Source: CAD feature listing. Evaluate the final solid. Frame: model axes, mm. A direction names the side the tool comes from. Give positions to 0.01 mm unless a question says otherwise; leave off trailing zeros. Order: outer loops, then holes, each group sorted by start corner. A loop starts at its lowest first (then second) coordinate and runs counter-clockwise, first axis right, second up. Notation, with made-up numbers: (43.5, 82) -> (78.5, 82) arc R18 ccw to (78.5, 100) -> close; hole circle Ø4 at (-27, 79.25). An arc over 180 degrees is marked (long way). Answer in a Markdown table with one row per item.
```python
from build123d import *

# Parameters (mm, degrees)
F0_R     = 38.1
F1_DEPTH = 25.4


with BuildPart() as f1:
    # F0 (on Front) → F1 (new body)
    with BuildSketch(Plane.XZ):
        with BuildLine():
            ThreePointArc((49.1988245643, 12.6536817364), (50.3981164721, 6.3772922205), (50.8, 0))
            ThreePointArc((50.8, 0), (50.3981164721, -6.3772922205), (49.1988245643, -12.6536817364))
            Line((49.1988245643, -12.6536817364), (49.5602090261, -13.2796179853))
            Line((49.5602090261, -13.2796179853), (72.5611820817, 0))
            Line((72.5611820817, 0), (49.5602090261, 13.2796179853))
            Line((49.5602090261, 13.2796179853), (49.1988245643, 12.6536817364))
        make_face()
        with BuildLine():
            ThreePointArc((48.9342727773, 13.641002447), (49.0690319755, 13.1480074912), (49.1988245643, 12.6536817364))
            Line((49.1988245643, 12.6536817364), (49.5602090261, 13.2796179853))
            Line((49.5602090261, 13.2796179853), (48.9342727773, 13.641002447))
        make_face()
        with BuildLine():
            Line((49.5602090261, -13.2796179853), (49.1988245643, -12.6536817364))
            ThreePointArc((49.1988245643, -12.6536817364), (49.0690319755, -13.1480074912), (48.9342727773, -13.641002447))
            Line((48.9342727773, -13.641002447), (49.5602090261, -13.2796179853))
        make_face()
        with BuildLine():
            ThreePointArc((36.2805910408, 35.5578221173), (43.9940905122, 25.4), (48.9342727773, 13.641002447))
            Line((48.9342727773, 13.641002447), (49.5602090261, 13.2796179853))
            Line((49.5602090261, 13.2796179853), (62.8398270114, 36.2805910408))
            Line((62.8398270114, 36.2805910408), (36.2805910408, 36.2805910408))
            Line((36.2805910408, 36.2805910408), (36.2805910408, 35.5578221173))
        make_face()
        with BuildLine():
            Line((49.5602090261, -13.2796179853), (48.9342727773, -13.641002447))
            ThreePointArc((48.9342727773, -13.641002447), (43.9940905122, -25.4), (36.2805910408, -35.5578221173))
            Line((36.2805910408, -35.5578221173), (36.2805910408, -36.2805910408))
            Line((36.2805910408, -36.2805910408), (62.8398270114, -36.2805910408))
            Line((62.8398270114, -36.2805910408), (49.5602090261, -13.2796179853))
        make_face()
        with BuildLine():
            ThreePointArc((35.5578221173, 36.2805910408), (35.9210244843, 35.9210244843), (36.2805910408, 35.5578221173))
            Line((36.2805910408, 35.5578221173), (36.2805910408, 36.2805910408))
            Line((36.2805910408, 36.2805910408), (35.5578221173, 36.2805910408))
        make_face()
        with BuildLine():
            Line((36.2805910408, -36.2805910408), (36.2805910408, -35.5578221173))
            ThreePointArc((36.2805910408, -35.5578221173), (35.9210244843, -35.9210244843), (35.5578221173, -36.2805910408))
            Line((35.5578221173, -36.2805910408), (36.2805910408, -36.2805910408))
        make_face()
        with BuildLine():
            ThreePointArc((13.641002447, 48.9342727773), (25.4, 43.9940905122), (35.5578221173, 36.2805910408))
            Line((35.5578221173, 36.2805910408), (36.2805910408, 36.2805910408))
            Line((36.2805910408, 36.2805910408), (36.2805910408, 62.8398270114))
            Line((36.2805910408, 62.8398270114), (13.2796179853, 49.5602090261))
            Line((13.2796179853, 49.5602090261), (13.641002447, 48.9342727773))
        make_face()
        with BuildLine():
            Line((36.2805910408, -36.2805910408), (35.5578221173, -36.2805910408))
            ThreePointArc((35.5578221173, -36.2805910408), (25.4, -43.9940905122), (13.641002447, -48.9342727773))
            Line((13.641002447, -48.9342727773), (13.2796179853, -49.5602090261))
            Line((13.2796179853, -49.5602090261), (36.2805910408, -62.8398270114))
            Line((36.2805910408, -62.8398270114), (36.2805910408, -36.2805910408))
        make_face()
        with BuildLine():
            ThreePointArc((12.6536817364, 49.1988245643), (13.1480074912, 49.0690319755), (13.641002447, 48.9342727773))
            Line((13.641002447, 48.9342727773), (13.2796179853, 49.5602090261))
            Line((13.2796179853, 49.5602090261), (12.6536817364, 49.1988245643))
        make_face()
        with BuildLine():
            Line((13.2796179853, -49.5602090261), (13.641002447, -48.9342727773))
            ThreePointArc((13.641002447, -48.9342727773), (13.1480074912, -49.0690319755), (12.6536817364, -49.1988245643))
            Line((12.6536817364, -49.1988245643), (13.2796179853, -49.5602090261))
        make_face()
        with BuildLine():
            ThreePointArc((-12.6536817364, 49.1988245643), (0, 50.8), (12.6536817364, 49.1988245643))
            Line((12.6536817364, 49.1988245643), (13.2796179853, 49.5602090261))
            Line((13.2796179853, 49.5602090261), (0, 72.5611820817))
            Line((0, 72.5611820817), (-13.2796179853, 49.5602090261))
            Line((-13.2796179853, 49.5602090261), (-12.6536817364, 49.1988245643))
        make_face()
        with BuildLine():
            Line((13.2796179853, -49.5602090261), (12.6536817364, -49.1988245643))
            ThreePointArc((12.6536817364, -49.1988245643), (0, -50.8), (-12.6536817364, -49.1988245643))
            Line((-12.6536817364, -49.1988245643), (-13.2796179853, -49.5602090261))
            Line((-13.2796179853, -49.5602090261), (0, -72.5611820817))
            Line((0, -72.5611820817), (13.2796179853, -49.5602090261))
        make_face()
        with BuildLine():
            ThreePointArc((-13.641002447, 48.9342727773), (-13.1480074912, 49.0690319755), (-12.6536817364, 49.1988245643))
            Line((-12.6536817364, 49.1988245643), (-13.2796179853, 49.5602090261))
            Line((-13.2796179853, 49.5602090261), (-13.641002447, 48.9342727773))
        make_face()
        with BuildLine():
            Line((-13.2796179853, -49.5602090261), (-12.6536817364, -49.1988245643))
            ThreePointArc((-12.6536817364, -49.1988245643), (-13.1480074912, -49.0690319755), (-13.641002447, -48.9342727773))
            Line((-13.641002447, -48.9342727773), (-13.2796179853, -49.5602090261))
        make_face()
        with BuildLine():
            ThreePointArc((-35.5578221173, 36.2805910408), (-25.4, 43.9940905122), (-13.641002447, 48.9342727773))
            Line((-13.641002447, 48.9342727773), (-13.2796179853, 49.5602090261))
            Line((-13.2796179853, 49.5602090261), (-36.2805910408, 62.8398270114))
            Line((-36.2805910408, 62.8398270114), (-36.2805910408, 36.2805910408))
            Line((-36.2805910408, 36.2805910408), (-35.5578221173, 36.2805910408))
        make_face()
        with BuildLine():
            Line((-13.2796179853, -49.5602090261), (-13.641002447, -48.9342727773))
            ThreePointArc((-13.641002447, -48.9342727773), (-25.4, -43.9940905122), (-35.5578221173, -36.2805910408))
            Line((-35.5578221173, -36.2805910408), (-36.2805910408, -36.2805910408))
            Line((-36.2805910408, -36.2805910408), (-36.2805910408, -62.8398270114))
            Line((-36.2805910408, -62.8398270114), (-13.2796179853, -49.5602090261))
        make_face()
        with BuildLine():
            ThreePointArc((-36.2805910408, 35.5578221173), (-35.9210244843, 35.9210244843), (-35.5578221173, 36.2805910408))
            Line((-35.5578221173, 36.2805910408), (-36.2805910408, 36.2805910408))
            Line((-36.2805910408, 36.2805910408), (-36.2805910408, 35.5578221173))
        make_face()
        with BuildLine():
            Line((-36.2805910408, -36.2805910408), (-35.5578221173, -36.2805910408))
            ThreePointArc((-35.5578221173, -36.2805910408), (-35.9210244843, -35.9210244843), (-36.2805910408, -35.5578221173))
            Line((-36.2805910408, -35.5578221173), (-36.2805910408, -36.2805910408))
        make_face()
        with BuildLine():
            ThreePointArc((-48.9342727773, 13.641002447), (-43.9940905122, 25.4), (-36.2805910408, 35.5578221173))
            Line((-36.2805910408, 35.5578221173), (-36.2805910408, 36.2805910408))
            Line((-36.2805910408, 36.2805910408), (-62.8398270114, 36.2805910408))
            Line((-62.8398270114, 36.2805910408), (-49.5602090261, 13.2796179853))
            Line((-49.5602090261, 13.2796179853), (-48.9342727773, 13.641002447))
        make_face()
        with BuildLine():
            Line((-36.2805910408, -36.2805910408), (-36.2805910408, -35.5578221173))
            ThreePointArc((-36.2805910408, -35.5578221173), (-43.9940905122, -25.4), (-48.9342727773, -13.641002447))
            Line((-48.9342727773, -13.641002447), (-49.5602090261, -13.2796179853))
            Line((-49.5602090261, -13.2796179853), (-62.8398270114, -36.2805910408))
            Line((-62.8398270114, -36.2805910408), (-36.2805910408, -36.2805910408))
        make_face()
        with BuildLine():
            ThreePointArc((-49.1988245643, 12.6536817364), (-49.0690319755, 13.1480074912), (-48.9342727773, 13.641002447))
            Line((-48.9342727773, 13.641002447), (-49.5602090261, 13.2796179853))
            Line((-49.5602090261, 13.2796179853), (-49.1988245643, 12.6536817364))
        make_face()
        with BuildLine():
            Line((-49.5602090261, -13.2796179853), (-48.9342727773, -13.641002447))
            ThreePointArc((-48.9342727773, -13.641002447), (-49.0690319755, -13.1480074912), (-49.1988245643, -12.6536817364))
            Line((-49.1988245643, -12.6536817364), (-49.5602090261, -13.2796179853))
        make_face()
        with BuildLine():
            ThreePointArc((-49.1988245643, -12.6536817364), (-50.8, 0), (-49.1988245643, 12.6536817364))
            Line((-49.1988245643, 12.6536817364), (-49.5602090261, 13.2796179853))
            Line((-49.5602090261, 13.2796179853), (-72.5611820817, 0))
            Line((-72.5611820817, 0), (-49.5602090261, -13.2796179853))
            Line((-49.5602090261, -13.2796179853), (-49.1988245643, -12.6536817364))
        make_face()
        with BuildLine():
            ThreePointArc((49.1988245643, -12.6536817364), (50.3981164721, -6.3772922205), (50.8, 0))
            ThreePointArc((50.8, 0), (50.3981164721, 6.3772922205), (49.1988245643, 12.6536817364))
            ThreePointArc((49.1988245643, 12.6536817364), (49.0690319755, 13.1480074912), (48.9342727773, 13.641002447))
            ThreePointArc((48.9342727773, 13.641002447), (43.9940905122, 25.4), (36.2805910408, 35.5578221173))
            ThreePointArc((36.2805910408, 35.5578221173), (35.9210244843, 35.9210244843), (35.5578221173, 36.2805910408))
            ThreePointArc((35.5578221173, 36.2805910408), (25.4, 43.9940905122), (13.641002447, 48.9342727773))
            ThreePointArc((13.641002447, 48.9342727773), (13.1480074912, 49.0690319755), (12.6536817364, 49.1988245643))
            ThreePointArc((12.6536817364, 49.1988245643), (0, 50.8), (-12.6536817364, 49.1988245643))
            ThreePointArc((-12.6536817364, 49.1988245643), (-13.1480074912, 49.0690319755), (-13.641002447, 48.9342727773))
            ThreePointArc((-13.641002447, 48.9342727773), (-25.4, 43.9940905122), (-35.5578221173, 36.2805910408))
            ThreePointArc((-35.5578221173, 36.2805910408), (-35.9210244843, 35.9210244843), (-36.2805910408, 35.5578221173))
            ThreePointArc((-36.2805910408, 35.5578221173), (-43.9940905122, 25.4), (-48.9342727773, 13.641002447))
            ThreePointArc((-48.9342727773, 13.641002447), (-49.0690319755, 13.1480074912), (-49.1988245643, 12.6536817364))
            ThreePointArc((-49.1988245643, 12.6536817364), (-50.8, 0), (-49.1988245643, -12.6536817364))
            ThreePointArc((-49.1988245643, -12.6536817364), (-49.0690319755, -13.1480074912), (-48.9342727773, -13.641002447))
            ThreePointArc((-48.9342727773, -13.641002447), (-43.9940905122, -25.4), (-36.2805910408, -35.5578221173))
            ThreePointArc((-36.2805910408, -35.5578221173), (-35.9210244843, -35.9210244843), (-35.5578221173, -36.2805910408))
            ThreePointArc((-35.5578221173, -36.2805910408), (-25.4, -43.9940905122), (-13.641002447, -48.9342727773))
            ThreePointArc((-13.641002447, -48.9342727773), (-13.1480074912, -49.0690319755), (-12.6536817364, -49.1988245643))
            ThreePointArc((-12.6536817364, -49.1988245643), (0, -50.8), (12.6536817364, -49.1988245643))
            ThreePointArc((12.6536817364, -49.1988245643), (13.1480074912, -49.0690319755), (13.641002447, -48.9342727773))
            ThreePointArc((13.641002447, -48.9342727773), (25.4, -43.9940905122), (35.5578221173, -36.2805910408))
            ThreePointArc((35.5578221173, -36.2805910408), (35.9210244843, -35.9210244843), (36.2805910408, -35.5578221173))
            ThreePointArc((36.2805910408, -35.5578221173), (43.9940905122, -25.4), (48.9342727773, -13.641002447))
            ThreePointArc((48.9342727773, -13.641002447), (49.0690319755, -13.1480074912), (49.1988245643, -12.6536817364))
        make_face()
        Circle(F0_R, mode=Mode.SUBTRACT)
    extrude(amount=F1_DEPTH)


solid = f1.part
```
(1) Access query for faces 1 (the flat face through (56.293, -12.522, -24.941)), 2 (the flat face through (24.941, -12.522, 56.293)), 3 (the flat face through (49, -13, -36.281)). Directions: +Z, -Z, +X, -X, +Y, -Y. A direction counts if a zero-diameter tool reaches every point of the face in a straight line with its end or side. Return the directions, or none.
A:
| item | result |
|---|---|
| face 1 | +X, +Y, -Y |
| face 2 | +Z, +Y, -Y |
| face 3 | -Z, +X, +Y, -Y |
(2) First-contact query: pin 1 Ø8 at (x, y) = (-53.5, -8) entering from +Z; pin 2 Ø8 at (x, y) = (21, -8) entering from -Z; pin 3 Ø12 at (y, z) = (-12, -6.5) entering from +X; pin 4 Ø1 at (x, z) = (-50.5, 37) entering from +Y. Flat tips, straight axial feed; report the tip coordinate or a pass-through.
A:
| item | result |
|---|---|
| pin 1 | stops at z = 36.28 |
| pin 2 | stops at z = -56.33 |
| pin 3 | stops at x = 71.7 |
| pin 4 | passes through |
(3) Section query B-B (z = 24). Return the cut outline in (x, y).
A:
| item | result |
|---|---|
| outline | (-55.75, -25.4) -> (-29.59, -25.4) -> (-29.59, 0) -> (-55.75, 0) -> close; (29.59, -25.4) -> (55.75, -25.4) -> (55.75, 0) -> (29.59, 0) -> close |
(4) Section query A-A (y = -18.25). Return the cut outline in (x, z), plus the area to 3 significant figures.
A:
| item | result |
|---|---|
| outline | (-72.56, 0) -> (-49.56, -13.28) -> (-62.84, -36.28) -> (-36.28, -36.28) -> (-36.28, -62.84) -> (-13.28, -49.56) -> (0, -72.56) -> (13.28, -49.56) -> (36.28, -62.84) -> (36.28, -36.28) -> (62.84, -36.28) -> (49.56, -13.28) -> (72.56, 0) -> (49.56, 13.28) -> (62.84, 36.28) -> (36.28, 36.28) -> (36.28, 62.84) -> (13.28, 49.56) -> (0, 72.56) -> (-13.28, 49.56) -> (-36.28, 62.84) -> (-36.28, 36.28) -> (-62.84, 36.28) -> (-49.56, 13.28) -> close; hole circle Ø76.2 at (0, 0) |
| area | 7,000 mm^2 |
(5) Pull-direction query (X, two-part tool) for faces 4 (the flat face through (-56.293, -12.522, 24.941)), 5 (the flat face through (6.55, -12.52, -61.22)), 6 (the flat face through (61.22, -12.52, 6.55)); classes: +X half, -X half, draft (parallel to the pull), parting line (faces both ways), or undercut.
A:
| item | result |
|---|---|
| face 4 | -X half |
| face 5 | undercut |
| face 6 | +X half |
(6) Section query C-C (x = -20.5). Return the cut outline in (y, z).
A:
| item | result |
|---|---|
| outline | (-25.4, -53.73) -> (0, -53.73) -> (0, -32.11) -> (-25.4, -32.11) -> close; (-25.4, 32.11) -> (0, 32.11) -> (0, 53.73) -> (-25.4, 53.73) -> close |
(7) Ray query, probe 1 along Z at (x, y) = (0, -12.5); probe 2 along X at (y, z) = (-2, 51); probe 3 along Z at (x, y) = (-26, -8.5). Return the intervals inside material, ascending.
A:
| item | result |
|---|---|
| probe 1 | z = -72.56 to -38.1, 38.1 to 72.56 |
| probe 2 | x = -36.28 to -15.77, -12.45 to 12.45, 15.77 to 36.28 |
| probe 3 | z = -56.9 to -27.85, 27.85 to 56.9 |
(8) Section query D-D (z = 53). Return the cut outline in (x, y), plus the area to 3 significant figures.
A:
| item | result |
|---|---|
| outline | (-36.28, -25.4) -> (-19.24, -25.4) -> (-19.24, 0) -> (-36.28, 0) -> close; (-11.29, -25.4) -> (11.29, -25.4) -> (11.29, 0) -> (-11.29, 0) -> close; (19.24, -25.4) -> (36.28, -25.4) -> (36.28, 0) -> (19.24, 0) -> close |
| area | 1,440 mm^2 |
